Verification items for the finished model (mm, model axes). A direction names the side the tool comes from. Round coordinates to 2 decimals unless told otherwise and drop trailing zeros. Loops run counter-clockwise (first coordinate to the right, second up) from the corner with the lowest first, then second, coordinate; pieces in that order, holes last. Notation, with made-up numbers: M 19,-20.75 L 58,-20.75 A17 cw 58,-2.75 Z; hole C -6,-34 d5. An arc over 180 degrees is marked long. One line per item, written item: value.
from build123d import *

# Parameters (mm, degrees)
SKETCH1_W               = 80
SKETCH1_H               = 40
BOSS_EXTRUDE1_DEPTH     = 20.5
SKETCH2_W               = 66.73316624
SKETCH2_H               = 22.854
CUT_EXTRUDE1_DEPTH      = 21.5
SKETCH3_W               = 30
SKETCH3_H               = 40
BOSS_EXTRUDE2_DEPTH     = 3.81
SKETCH4_R               = 4
CUT_EXTRUDE2_DEPTH      = 5.87375
SKETCH6_W               = 66.73316624
SKETCH6_H               = 10
CUT_EXTRUDE4_DEPTH      = 32.427
CUT_EXTRUDE4_DEPTH_BACK = 9.573
FILLET4_R               = 2.54
CUT_EXTRUDE5_DEPTH      = 5.25
BOSS_EXTRUDE3_DEPTH     = 5.87375
BOSS_EXTRUDE4_DEPTH     = 5.87375
CUT_EXTRUDE6_DEPTH      = 2.823417
CUT_EXTRUDE7_DEPTH      = 2.823417
BOSS_EXTRUDE5_DEPTH     = 0.508
BOSS_EXTRUDE6_DEPTH     = 0.508


with BuildPart() as part:
    # Sketch1 → Boss-Extrude1 (new body)
    with BuildSketch(Plane.XY):
        Rectangle(SKETCH1_W, SKETCH1_H)
    extrude(amount=BOSS_EXTRUDE1_DEPTH)

    # Sketch2 → Cut-Extrude1 (cut, through all)
    with BuildSketch(Plane.XY.offset(20.5)):
        Rectangle(SKETCH2_W, SKETCH2_H)
    extrude(amount=-CUT_EXTRUDE1_DEPTH, mode=Mode.SUBTRACT)

    # Sketch3 → Boss-Extrude2 (add, symmetric)
    with BuildSketch(Plane(origin=(40, 0, 0), x_dir=(0, 0, -1), z_dir=(1, 0, 0))):
        with Locations((-10.25, 0)):
            Rectangle(SKETCH3_W, SKETCH3_H)
    boss_extrude2 = extrude(amount=BOSS_EXTRUDE2_DEPTH, both=True)

    # Mirror1: Boss-Extrude2 across plane
    add(boss_extrude2.mirror(Plane(origin=(0, 0, 0), x_dir=(0, 0, 1), z_dir=(1, 0, 0))))

    # Sketch4 → Cut-Extrude2 (cut)
    with BuildSketch(Plane(origin=(43.81, 0, 0), x_dir=(0, 0, -1), z_dir=(1, 0, 0))):
        with Locations((-10.25, 0)):
            Circle(SKETCH4_R)
    cut_extrude2 = extrude(amount=-CUT_EXTRUDE2_DEPTH, mode=Mode.SUBTRACT)

    # Mirror2: Cut-Extrude2 across plane
    add(cut_extrude2.mirror(Plane(origin=(0, 0, 0), x_dir=(0, 0, 1), z_dir=(1, 0, 0))), mode=Mode.SUBTRACT)

    # Sketch6 → Cut-Extrude4 (cut, two sides)
    with BuildSketch(Plane(origin=(0, -11.427, 0), x_dir=(1, 0, 0), z_dir=(0, 1, 0))) as cut_extrude4_sk:
        with Locations((0, -10.25)):
            Rectangle(SKETCH6_W, SKETCH6_H)
    extrude(amount=CUT_EXTRUDE4_DEPTH, mode=Mode.SUBTRACT)
    extrude(cut_extrude4_sk.sketch, amount=-CUT_EXTRUDE4_DEPTH_BACK, mode=Mode.SUBTRACT)

    # Fillet4
    fillet4_edges = [part.edges().sort_by_distance(p)[0] for p in [
        (40, 20, 25.25),
        (40, -20, 25.25),
        (40, -20, -4.75),
        (40, 20, -4.75),
        (-40, -20, 25.25),
        (-40, 20, 25.25),
        (-40, 20, -4.75),
        (-40, -20, -4.75),
    ]]
    fillet(fillet4_edges, radius=FILLET4_R)

    # Sketch7 → Cut-Extrude5 (cut)
    with BuildSketch(Plane(origin=(0, 0, 0), x_dir=(-1, 0, 0), z_dir=(0, 0, -1))):
        with BuildLine():
            Line((-32.5, 15.016), (32.5, 15.016))
            ThreePointArc((32.5, 15.016), (33.516, 14), (32.5, 12.984))
            Line((32.5, 12.984), (-32.5, 12.984))
            ThreePointArc((-32.5, 12.984), (-33.516, 14), (-32.5, 15.016))
        make_face()
    cut_extrude5 = extrude(amount=-CUT_EXTRUDE5_DEPTH, mode=Mode.SUBTRACT)

    # Mirror3: Cut-Extrude5 across plane
    add(cut_extrude5.mirror(Plane.ZX), mode=Mode.SUBTRACT)

    # Sketch8 → Boss-Extrude3 (add)
    with BuildSketch(Plane(origin=(43.81, 0, 0), x_dir=(0, 0, -1), z_dir=(1, 0, 0))):
        with BuildLine():
            Line((-13.340048543, 2.54), (-13.340048543, -2.54))
            ThreePointArc((-13.340048543, -2.54), (-14.25, 0), (-13.340048543, 2.54))
        make_face()
    extrude(amount=-BOSS_EXTRUDE3_DEPTH)

    # Sketch9 → Boss-Extrude4 (add)
    with BuildSketch(Plane.ZY.offset(43.81)):
        with BuildLine():
            Line((13.340048543, 2.54), (13.340048543, -2.54))
            ThreePointArc((13.340048543, -2.54), (14.25, 0), (13.340048543, 2.54))
        make_face()
    extrude(amount=-BOSS_EXTRUDE4_DEPTH)

    # Sketch10 → Cut-Extrude6 (cut)
    with BuildSketch(Plane.ZY.offset(-33.36658312)):
        Polygon((20.5, 11.427), (15.25, 11.427), (15.25, 20), (5.25, 20), (5.25, 14.53036751), (5.25, 13.46963249), (5.25, 11.427), (0, 11.427), (0, -11.427), (5.25, -11.427), (5.25, -13.46963249), (5.25, -14.53036751), (5.25, -20), (15.25, -20), (15.25, -11.427), (20.5, -11.427), align=None)
    extrude(amount=-CUT_EXTRUDE6_DEPTH, mode=Mode.SUBTRACT)

    # Sketch11 → Cut-Extrude7 (cut)
    with BuildSketch(Plane(origin=(-33.36658312, 0, 0), x_dir=(0, 0, -1), z_dir=(1, 0, 0))):
        Polygon((-20.5, -11.427), (-15.25, -11.427), (-15.25, -20), (-5.25, -20), (-5.25, -14.53036751), (-5.25, -13.46963249), (-5.25, -11.427), (0, -11.427), (0, 11.427), (-5.25, 11.427), (-5.25, 13.46963249), (-5.25, 14.53036751), (-5.25, 20), (-15.25, 20), (-15.25, 11.427), (-20.5, 11.427), align=None)
    extrude(amount=-CUT_EXTRUDE7_DEPTH, mode=Mode.SUBTRACT)

    # Sketch12 → Boss-Extrude5 (add)
    with BuildSketch(Plane.ZY.offset(-36.19)):
        with BuildLine():
            Line((-4.75, 17.46), (-4.75, -17.46))
            ThreePointArc((-4.75, -17.46), (-4.006051224, -19.256051224), (-2.21, -20))
            Line((-2.21, -20), (0, -20))
            Line((0, -20), (0, -11.427))
            Line((0, -11.427), (5.25, -11.427))
            Line((5.25, -11.427), (5.25, -20))
            Line((5.25, -20), (15.25, -20))
            Line((15.25, -20), (15.25, -11.427))
            Line((15.25, -11.427), (20.5, -11.427))
            Line((20.5, -11.427), (20.5, -20))
            Line((20.5, -20), (22.71, -20))
            ThreePointArc((22.71, -20), (24.506051224, -19.256051224), (25.25, -17.46))
            Line((25.25, -17.46), (25.25, 17.46))
            ThreePointArc((25.25, 17.46), (24.506051224, 19.256051224), (22.71, 20))
            Line((22.71, 20), (20.5, 20))
            Line((20.5, 20), (20.5, 11.427))
            Line((20.5, 11.427), (15.25, 11.427))
            Line((15.25, 11.427), (15.25, 20))
            Line((15.25, 20), (5.25, 20))
            Line((5.25, 20), (5.25, 11.427))
            Line((5.25, 11.427), (0, 11.427))
            Line((0, 11.427), (0, 20))
            Line((0, 20), (-2.21, 20))
            ThreePointArc((-2.21, 20), (-4.006051224, 19.256051224), (-4.75, 17.46))
        make_face()
    extrude(amount=BOSS_EXTRUDE5_DEPTH)

    # Sketch13 → Boss-Extrude6 (add)
    with BuildSketch(Plane(origin=(-36.19, 0, 0), x_dir=(0, 0, -1), z_dir=(1, 0, 0))):
        with BuildLine():
            Line((0, -20), (2.21, -20))
            ThreePointArc((2.21, -20), (4.006051224, -19.256051224), (4.75, -17.46))
            Line((4.75, -17.46), (4.75, 17.46))
            ThreePointArc((4.75, 17.46), (4.006051224, 19.256051224), (2.21, 20))
            Line((2.21, 20), (0, 20))
            Line((0, 20), (0, 11.427))
            Line((0, 11.427), (-5.25, 11.427))
            Line((-5.25, 11.427), (-5.25, 20))
            Line((-5.25, 20), (-15.25, 20))
            Line((-15.25, 20), (-15.25, 11.427))
            Line((-15.25, 11.427), (-20.5, 11.427))
            Line((-20.5, 11.427), (-20.5, 20))
            Line((-20.5, 20), (-22.71, 20))
            ThreePointArc((-22.71, 20), (-24.506051224, 19.256051224), (-25.25, 17.46))
            Line((-25.25, 17.46), (-25.25, -17.46))
            ThreePointArc((-25.25, -17.46), (-24.506051224, -19.256051224), (-22.71, -20))
            Line((-22.71, -20), (-20.5, -20))
            Line((-20.5, -20), (-20.5, -11.427))
            Line((-20.5, -11.427), (-15.25, -11.427))
            Line((-15.25, -11.427), (-15.25, -20))
            Line((-15.25, -20), (-5.25, -20))
            Line((-5.25, -20), (-5.25, -11.427))
            Line((-5.25, -11.427), (0, -11.427))
            Line((0, -11.427), (0, -20))
        make_face()
    extrude(amount=BOSS_EXTRUDE6_DEPTH)


solid = part.part
(1) Thickness scan on L1, parallel to Y at x = -23.5, z = 3; L2, parallel to X at y = -8, z = 0.5; L3, parallel to X at y = -3.5, z = 9.75. Record the ranges inside material, lowest first. Write a range as from..to.
Completed:
L1: y = -20..-15.02, -12.98..-11.43, 11.43..12.98, 15.02..20
L2: x = -43.81..-35.68, 35.68..43.81
L3: x = -37.94..-35.68, 35.68..37.94
(2) Sectioned sample at B-B on z = 10.25. Enter the section's corners in (x, y).
Completed:
outline: M -43.81,-20 L -35.68,-20 L -35.68,20 L -43.81,20 L -43.81,4 L -37.94,4 L -37.94,-4 L -43.81,-4 Z; M 35.68,-20 L 43.81,-20 L 43.81,-4 L 37.94,-4 L 37.94,4 L 43.81,4 L 43.81,20 L 35.68,20 Z
(3) Tool access check on faces 4 (the face through (0, 12.984, 3)), 5 (the face through (0, -16, 5.25)), 6 (the face through (0, 16, 0)), 7 (the face through (0, 16, 20.5)), 8 (the face through (40.914, -0.137, 6.252)). Record the directions out of +Z, -Z, +X, -X, +Y, -Y that give a thin tool (end or side, any length) a straight path to the whole face; none if there is none.
Completed:
face 4: -Z
face 5: +Y, -Y
face 6: -Z, +Y, -Y
face 7: +Z, +Y, -Y
face 8: +X
(4) Depth check by flat-ended pin: pin 1 Ø10.5 at (y, z) = (0, 10.25) entering from +X; pin 2 Ø2.5 at (x, y) = (11, 15.5) entering from +Z; pin 3 Ø2.5 at (x, y) = (-3, 16.5) entering from -Z; pin 4 Ø10 at (x, y) = (-21, -4) entering from +Z. Enter the tip coordinate at first touch or a pass-through.
Completed:
pin 1: stops at x = 43.81
pin 2: stops at z = 20.5
pin 3: stops at z = 0
pin 4: passes through
(5) Sectioned sample at C-C on y = 0. Enter the section's corners in (x, z).
Completed:
outline: M -43.81,-4.75 L -35.68,-4.75 L -35.68,25.25 L -43.81,25.25 L -43.81,13.34 L -37.94,13.34 L -37.94,6.25 L -43.81,6.25 Z; M 35.68,-4.75 L 43.81,-4.75 L 43.81,6.25 L 37.94,6.25 L 37.94,13.34 L 43.81,13.34 L 43.81,25.25 L 35.68,25.25 Z
(6) Sectioned sample at A-A on x = -31.5. Enter the section's corners in (y, z).
Completed:
outline: M -20,0 L -15.02,0 L -15.02,5.25 L -20,5.25 Z; M -20,15.25 L -11.43,15.25 L -11.43,20.5 L -20,20.5 Z; M -12.98,0 L -11.43,0 L -11.43,5.25 L -12.98,5.25 Z; M 11.43,0 L 12.98,0 L 12.98,5.25 L 11.43,5.25 Z; M 11.43,15.25 L 20,15.25 L 20,20.5 L 11.43,20.5 Z; M 15.02,0 L 20,0 L 20,5.25 L 15.02,5.25 Z
(7) Sectioned sample at D-D on z = 19.5. Enter the section's corners in (x, y).
Completed:
outline: M -43.81,-20 L 43.81,-20 L 43.81,20 L -43.81,20 Z; hole M -35.68,-11.43 L 35.68,-11.43 L 35.68,11.43 L -35.68,11.43 Z
(8) Mould release check, pull along X, two halves, no side actions. Record for faces 1 (the face through (-37.936, 0, 10)), 2 (the face through (33.516, -13.978, 2.588)), 3 (the face through (-40.914, -0.137, 6.252)): +X half, -X half, draft (parallel to the pull), parting line (faces both ways), or undercut.
Completed:
face 1: -X half
face 2: undercut
face 3: draft
